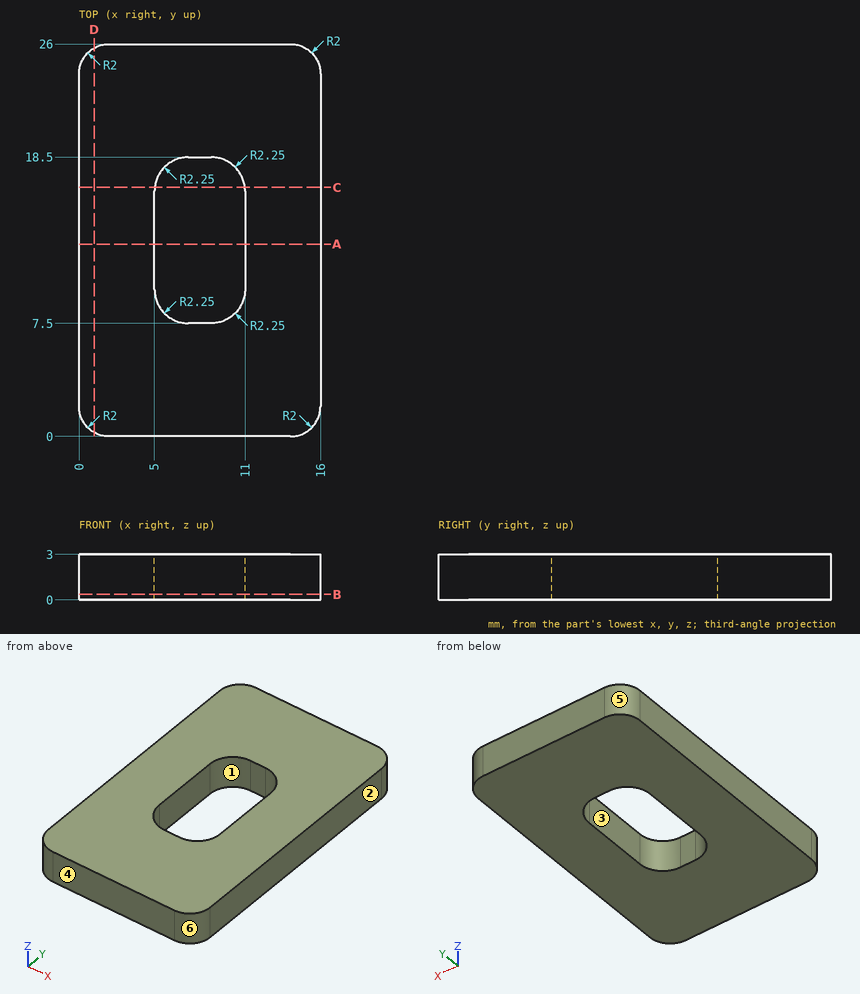
Input: dimensioned drawing with shaded views. Units: mm. Origin: part minimum x, y, z. A direction names the side the tool comes from. Round coordinates to 2 decimals unless told otherwise and drop trailing zeros. Order: outer loops, then holes, each group sorted by start corner. A loop starts at its lowest first (then second) coordinate and runs counter-clockwise, first axis right, second up. Notation, with made-up numbers: (-36.5, -32.75) - (16.5, -32.75) arc R3 cw to (16.5, -28.75) - close; hole circle Ø11 at (3.25, 36). An arc over 180 degrees is marked (long way). Answer as a JSON object with one key per item and string values. Group by question number.
(1) Draft query along X for the marked faces 3, 4, 5 and 6. Return one class per face: released by +X, released by -X, zero draft, split by the parting line, or undercut.
(2) Cut plane C-C (y = 16.5). Return loops of the section in (x, z).
(3) Reachability of the marked faces 1 and 2 from +Z, -Z, +X, -X, +Y, -Y: full face, straight path, thin tool, end or side. Return the list, or none.
(4) Cut plane B-B (z = 0.35). Return loops of the section in (x, y).
(5) Cut plane A-A (y = 12.75). Return loops of the section in (x, z).
(6) Cut plane D-D (x = 1). Return loops of the section in (y, z).
(7) Material intervals for probe 1 along Y at (x, z) = (8.5, 1.05); probe 2 along X at (y, z) = (14.75, 2.55); probe 3 along Y at (x, z) = (9.25, 2.35), sorted ascending. Write a range as from..to.
Here are the results:
{
 "1": {"face 3": "undercut", "face 4": "zero draft", "face 5": "released by -X", "face 6": "released by +X"},
 "2": {"outline": "(0, 0) - (5.01, 0) - (5.01, 3) - (0, 3) - close; (10.99, 0) - (16, 0) - (16, 3) - (10.99, 3) - close"},
 "3": {"face 1": "+Z, -Z", "face 2": "+Z, -Z, +X, +Y, -Y"},
 "4": {"outline": "(0, 2) arc R2 ccw to (2, 0) - (14, 0) arc R2 ccw to (16, 2) - (16, 24) arc R2 ccw to (14, 26) - (2, 26) arc R2 ccw to (0, 24) - close; hole (5, 9.75) arc R2.25 ccw to (7.25, 7.5) - (8.75, 7.5) arc R2.25 ccw to (11, 9.75) - (11, 16.25) arc R2.25 ccw to (8.75, 18.5) - (7.25, 18.5) arc R2.25 ccw to (5, 16.25) - close"},
 "5": {"outline": "(0, 0) - (5, 0) - (5, 3) - (0, 3) - close; (11, 0) - (16, 0) - (16, 3) - (11, 3) - close"},
 "6": {"outline": "(0.27, 0) - (25.73, 0) - (25.73, 3) - (0.27, 3) - close"},
 "7": {"probe 1": "y = 0..7.5, 18.5..26", "probe 2": "x = 0..5, 11..16", "probe 3": "y = 0..7.56, 18.44..26"}
}
